```python
from build123d import *

# Parameters (mm, degrees)
SKETCH1_R           = 5
BRANCH_DEPTH        = 120
BOSS_EXTRUDE1_DEPTH = 7.5
SKETCH3_W           = 100
SKETCH3_H           = 80
BOSS_EXTRUDE2_DEPTH = 7.5


with BuildPart() as part:
    # Sketch1 → branch (new body)
    with BuildSketch(Plane(origin=(0, 0, 0), x_dir=(1, 0, 0), z_dir=(0, 1, 0))):
        with Locations(Location((0, 0, 0), (0, 0, 270))):
            Circle(SKETCH1_R)
    extrude(amount=BRANCH_DEPTH)

    # Sketch2 → Boss-Extrude1 (add)
    with BuildSketch(Plane(origin=(0, 120, 0), x_dir=(1, 0, 0), z_dir=(0, 1, 0))):
        with BuildLine():
            Line((-5, 0), (-5, -120))
            Line((-5, -120), (5, -120))
            Line((5, -120), (5, 0))
            ThreePointArc((5, 0), (0, 5), (-5, 0))
        make_face()
    extrude(amount=BOSS_EXTRUDE1_DEPTH)

    # Sketch3 → Boss-Extrude2 (add)
    with BuildSketch(Plane.XY.offset(120)):
        with Locations((0, 160)):
            Rectangle(SKETCH3_W, SKETCH3_H)
    extrude(amount=-BOSS_EXTRUDE2_DEPTH)


solid = part.part
```
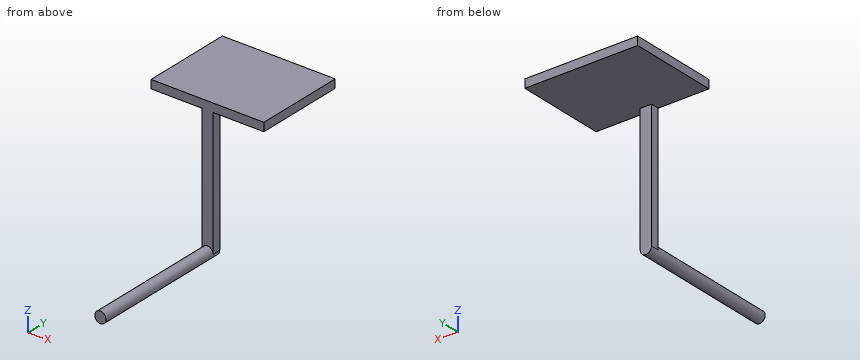
The model under review builds one solid part; all positions refer to its coordinate system, in mm. Round coordinates to 2 decimals unless told otherwise and drop trailing zeros. Loops run counter-clockwise (first coordinate to the right, second up) from the corner with the lowest first, then second, coordinate; pieces in that order, holes last.
1) Wall thickness on line 1 along Y through (x, z) = (-3, 40); line 2 along Y through (x, z) = (44, 113.5); line 3 along Z through (x, y) = (-43, 177): over which ranges is each line inside the solid? List them lowest first.
Values follow:
line 1: y = 120 to 127.5
line 2: y = 120 to 200
line 3: z = 112.5 to 120
2) Consider section C-C on z = 70.5. State the section outline as (x, y) points, then the cut area to 3 significant figures.
Values follow:
outline: (-5, 120) - (5, 120) - (5, 127.5) - (-5, 127.5) - close
area: 75.0 mm2
3) Consider section D-D on x = 18.5. State the section outline as (y, z) points.
Values follow:
outline: (120, 112.5) - (200, 112.5) - (200, 120) - (120, 120) - close
4) Clearance check with flat-ended pins moving along their axes: P1, Ø24, axis at x = -14, y = 163.5, coming from the -Z side; P2, Ø4, axis at y = 124.5, z = 33.5, coming from the -X side; P3, Ø8, axis at x = 0, z = 48, coming from the +Y side. State where each tip first meets the part, or that it passes through.
Values follow:
P1: stops at z = 112.5
P2: stops at x = -5
P3: stops at y = 127.5
5) Consider section B-B on y = 64. State the section outline as (x, z) points.
Values follow:
outline: circle Ø10 at (0, 0)
6) Consider section A-A on x = 0. State the section outline as (y, z) points.
Values follow:
outline: (0, -5) - (127.5, -5) - (127.5, 112.5) - (200, 112.5) - (200, 120) - (120, 120) - (120, 5) - (0, 5) - close
